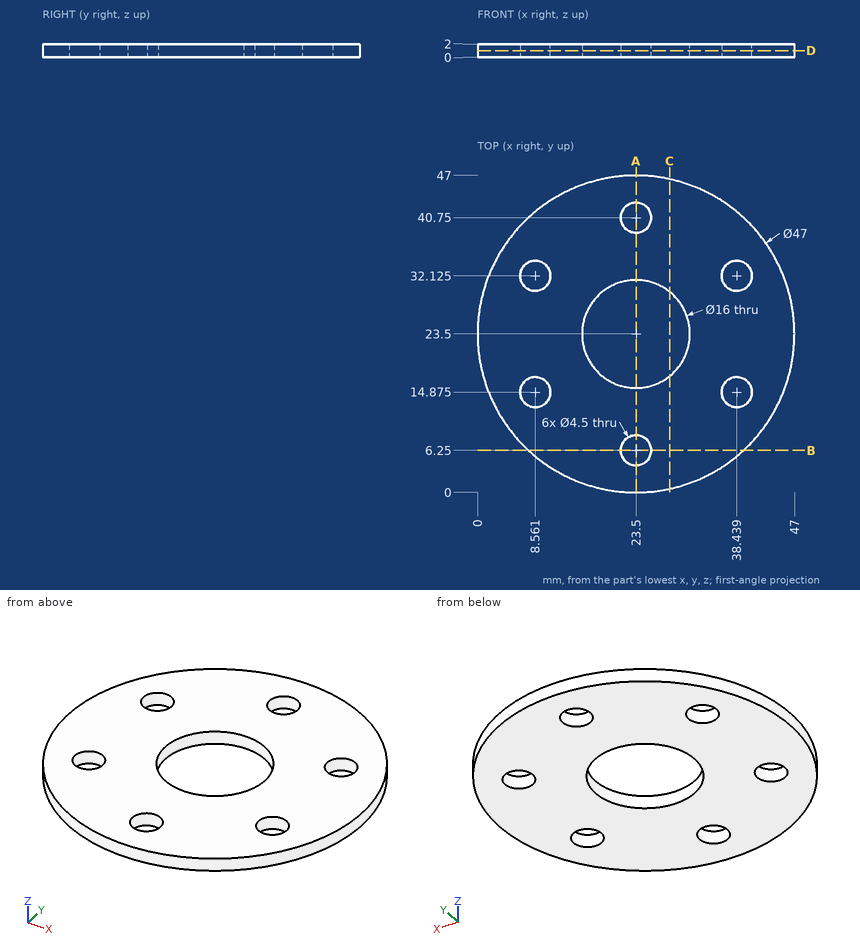
Geometry check sheet. Reference: drawing and pictorial views, mm from the part's lowest x, y, z. Give positions to 0.01 mm unless a question says otherwise; leave off trailing zeros. Order: outer loops, then holes, each group sorted by start corner. A loop starts at its lowest first (then second) coordinate and runs counter-clockwise, first axis right, second up. Notation, with made-up numbers: M 52.25,75 L 72.25,75 A19 cw 72.25,104 Z; hole C -28.5,7 d1. An arc over 180 degrees is marked long. Answer in a Markdown table with one row per item.
1) Cross-section at C-C, the plane x = 28.5. Enter the section's corners in (y, z) (3 decimals).
Filled sheet:
| item | result |
|---|---|
| outline | M 0.538,0 L 17.255,0 L 17.255,2 L 0.538,2 Z; M 29.745,0 L 46.462,0 L 46.462,2 L 29.745,2 Z |
2) Cross-section at B-B, the plane y = 6.25. Enter the section's corners in (x, z), plus the area to 3 significant figures.
Filled sheet:
| item | result |
|---|---|
| outline | M 7.54,0 L 21.25,0 L 21.25,2 L 7.54,2 Z; M 25.75,0 L 39.46,0 L 39.46,2 L 25.75,2 Z |
| area | 54.8 mm2 |
3) Cross-section at A-A, the plane x = 23.5. Enter the section's corners in (y, z), plus the area to 3 significant figures.
Filled sheet:
| item | result |
|---|---|
| outline | M 0,0 L 4,0 L 4,2 L 0,2 Z; M 8.5,0 L 15.5,0 L 15.5,2 L 8.5,2 Z; M 31.5,0 L 38.5,0 L 38.5,2 L 31.5,2 Z; M 43,0 L 47,0 L 47,2 L 43,2 Z |
| area | 44.0 mm2 |
4) Cross-section at D-D, the plane z = 1. Enter the section's corners in (x, y) (3 decimals).
Filled sheet:
| item | result |
|---|---|
| outline | C 23.5,23.5 d47; hole C 8.561,14.875 d4.5; hole C 8.561,32.125 d4.5; hole C 23.5,23.5 d16; hole C 23.5,6.25 d4.5; hole C 23.5,40.75 d4.5; hole C 38.439,14.875 d4.5; hole C 38.439,32.125 d4.5 |
5) Gauge pin test, flat end, axial feed: P1, Ø1, axis at x = 29, z = 1.5, coming from the -Y side. Record the tip position at first contact, or that the pin passes through.
Filled sheet:
| item | result |
|---|---|
| P1 | stops at y = 0.54 |
6) Thickness scan on L1, parallel to Y at x = 23.5, z = 1.15; L2, parallel to Y at x = 39.5, z = 1.2; L3, parallel to Y at x = 7, z = 0.55 (1 decimal). Record the ranges inside material, lowest first. Write a range as [from, to].
Filled sheet:
| item | result |
|---|---|
| L1 | y = [0, 4], [8.5, 15.5], [31.5, 38.5], [43, 47] |
| L2 | y = [6.29, 12.89], [16.86, 30.14], [34.11, 40.71] |
| L3 | y = [6.8, 13.3], [16.5, 30.5], [33.7, 40.2] |
